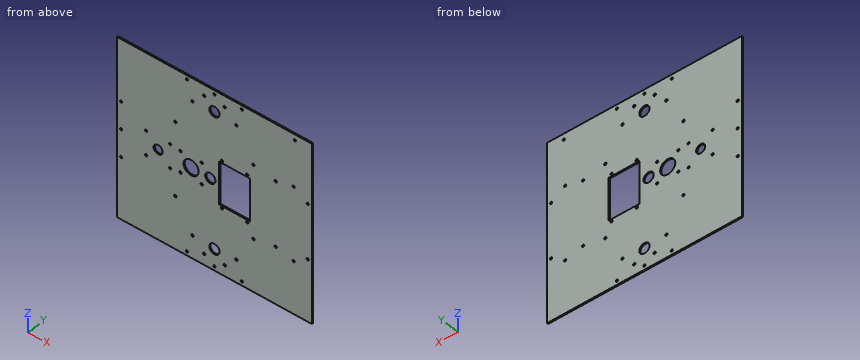
from build123d import *

# Parameters (mm, degrees)
SKETCH_1_W          = 284
SKETCH_1_H          = 260
EXTRUDE_1_DEPTH     = 2
SKETCH_2_R          = 6.65
SKETCH_2_R_2        = 1.6
SKETCH_2_R_3        = 11.05
SKETCH_2_R_4        = 1.75
SKETCH_2_R_5        = 1.65
SKETCH_2_W          = 45
SKETCH_2_H          = 62
CUT_EXTRUDE_1_DEPTH = 10
SKETCH_3_R          = 1.75
CUT_EXTRUDE_2_DEPTH = 10
SKETCH_4_R          = 7.5
CUT_EXTRUDE_3_DEPTH = 10
SKETCH_5_R          = 1.75
CUT_EXTRUDE_4_DEPTH = 4.5


with BuildPart() as part:
    # 草图1 → 凸台-拉伸1 (new body)
    with BuildSketch(Plane(origin=(0, 0, 0), x_dir=(1, 0, 0), z_dir=(0, 1, 0))):
        Rectangle(SKETCH_1_W, SKETCH_1_H)
    extrude(amount=EXTRUDE_1_DEPTH)

    # 草图2 → 切除-拉伸1 (cut)
    with BuildSketch(Plane(origin=(0, 2, 0), x_dir=(1, 0, 0), z_dir=(0, 1, 0))):
        with Locations(Location((-82, 0, 0), (0, 0, 270))):
            Circle(SKETCH_2_R)
        with Locations(Location((-99.536248173, 17.536248173, 0), (0, 0, 270))):
            Circle(SKETCH_2_R_2)
        with Locations(Location((-64.463751827, 17.536248173, 0), (0, 0, 270))):
            Circle(SKETCH_2_R_2)
        with Locations(Location((-64.463751827, -17.536248173, 0), (0, 0, 270))):
            Circle(SKETCH_2_R_2)
        with Locations(Location((-99.536248173, -17.536248173, 0), (0, 0, 270))):
            Circle(SKETCH_2_R_2)
        with Locations(Location((-34, 0, 0), (0, 0, 270))):
            Circle(SKETCH_2_R_3)
        with Locations(Location((-18.5, 15.5, 0), (0, 0, 270))):
            Circle(SKETCH_2_R_4)
        with Locations(Location((-18.5, -15.5, 0), (0, 0, 270))):
            Circle(SKETCH_2_R_4)
        with Locations(Location((-49.5, -15.5, 0), (0, 0, 270))):
            Circle(SKETCH_2_R_4)
        with Locations(Location((-49.5, 15.5, 0), (0, 0, 270))):
            Circle(SKETCH_2_R_4)
        with Locations(Location((-40, 124, 0), (0, 0, 270))):
            Circle(SKETCH_2_R_5)
        with Locations(Location((0, 124, 0), (0, 0, 270))):
            Circle(SKETCH_2_R_5)
        with Locations(Location((40, 124, 0), (0, 0, 270))):
            Circle(SKETCH_2_R_5)
        with Locations(Location((117.5, -121.5, 0), (0, 0, 270))):
            Circle(SKETCH_2_R_5)
        with Locations(Location((40, -124, 0), (0, 0, 270))):
            Circle(SKETCH_2_R_5)
        with Locations(Location((0, -124, 0), (0, 0, 270))):
            Circle(SKETCH_2_R_5)
        with Locations(Location((-40, -124, 0), (0, 0, 270))):
            Circle(SKETCH_2_R_5)
        with Locations(Location((-136, 40, 0), (0, 0, 270))):
            Circle(SKETCH_2_R_5)
        with Locations(Location((-136, -40, 0), (0, 0, 270))):
            Circle(SKETCH_2_R_5)
        with Locations(Location((-136, 0, 0), (0, 0, 270))):
            Circle(SKETCH_2_R_5)
        with Locations(Location((136, 40, 0), (0, 0, 270))):
            Circle(SKETCH_2_R_5)
        with Locations(Location((136, -40, 0), (0, 0, 270))):
            Circle(SKETCH_2_R_5)
        with Locations(Location((115.551101602, -53.6, 0), (0, 0, 270))):
            Circle(SKETCH_2_R_5)
        with Locations(Location((89.320585023, -47.2, 0), (0, 0, 270))):
            Circle(SKETCH_2_R_5)
        with Locations(Location((115.551101602, 53.6, 0), (0, 0, 270))):
            Circle(SKETCH_2_R_5)
        with Locations(Location((89.320585023, 47.2, 0), (0, 0, 270))):
            Circle(SKETCH_2_R_5)
        with Locations(Location((11.15, -34.2, 0), (0, 0, 270))):
            Circle(SKETCH_2_R_4)
        with Locations(Location((47.85, -34.2, 0), (0, 0, 270))):
            Circle(SKETCH_2_R_4)
        with Locations(Location((47.85, 34.2, 0), (0, 0, 270))):
            Circle(SKETCH_2_R_4)
        with Locations(Location((11.15, 34.2, 0), (0, 0, 270))):
            Circle(SKETCH_2_R_4)
        with Locations((29.5, 0)):
            Rectangle(SKETCH_2_W, SKETCH_2_H)
    extrude(amount=-CUT_EXTRUDE_1_DEPTH, mode=Mode.SUBTRACT)

    # 草图3 → 切除-拉伸2 (cut)
    with BuildSketch(Plane(origin=(0, 2, 0), x_dir=(1, 0, 0), z_dir=(0, 1, 0))):
        with Locations(Location((15, -114, 0), (0, 0, 270))):
            Circle(SKETCH_3_R)
        with Locations(Location((-15, -114, 0), (0, 0, 270))):
            Circle(SKETCH_3_R)
        with Locations(Location((15, 114, 0), (0, 0, 270))):
            Circle(SKETCH_3_R)
        with Locations(Location((-15, 114, 0), (0, 0, 270))):
            Circle(SKETCH_3_R)
    extrude(amount=-CUT_EXTRUDE_2_DEPTH, mode=Mode.SUBTRACT)

    # 草图4 → 切除-拉伸3 (cut)
    with BuildSketch(Plane(origin=(0, 2, 0), x_dir=(1, 0, 0), z_dir=(0, 1, 0))):
        with Locations(Location((-6, 0, 0), (0, 0, 270))):
            Circle(SKETCH_4_R)
        with Locations(Location((0, 99, 0), (0, 0, 270))):
            Circle(SKETCH_4_R)
        with Locations(Location((0, -99, 0), (0, 0, 270))):
            Circle(SKETCH_4_R)
    extrude(amount=-CUT_EXTRUDE_3_DEPTH, mode=Mode.SUBTRACT)

    # 草图5 → 切除-拉伸4 (cut)
    with BuildSketch(Plane(origin=(0, 2, 0), x_dir=(1, 0, 0), z_dir=(0, 1, 0))):
        with Locations(Location((57.002701991, 53.5, 0), (0, 0, 270))):
            Circle(SKETCH_5_R)
        with Locations(Location((32.002701991, 96.801270189, 0), (0, 0, 270))):
            Circle(SKETCH_5_R)
        with Locations(Location((-32.002701991, 96.801270189, 0), (0, 0, 270))):
            Circle(SKETCH_5_R)
        with Locations(Location((-57.002701991, 53.5, 0), (0, 0, 270))):
            Circle(SKETCH_5_R)
        with Locations(Location((-57.002701991, -53.5, 0), (0, 0, 270))):
            Circle(SKETCH_5_R)
        with Locations(Location((-32.002701991, -96.801270189, 0), (0, 0, 270))):
            Circle(SKETCH_5_R)
        with Locations(Location((32.002701991, -96.801270189, 0), (0, 0, 270))):
            Circle(SKETCH_5_R)
        with Locations(Location((57.002701991, -53.5, 0), (0, 0, 270))):
            Circle(SKETCH_5_R)
    extrude(amount=-CUT_EXTRUDE_4_DEPTH, mode=Mode.SUBTRACT)


solid = part.part
Source: CAD feature listing. Evaluate the final solid. Frame: model axes, mm. Round coordinates to 2 decimals unless told otherwise and drop trailing zeros. Order: outer loops, then holes, each group sorted by start corner. A loop starts at its lowest first (then second) coordinate and runs counter-clockwise, first axis right, second up. Notation, with made-up numbers: (67, 67) - (85, 67) arc R10 cw to (85, 74) - close; hole circle Ø10 at (85, 42). An arc over 180 degrees is marked (long way). Use a Markdown table: item, result. Add a question column.
1. Line query: probe 1 along Z at (x, y) = (31.5, 0.5); probe 2 along Z at (x, y) = (25, 1.2); probe 3 along X at (y, z) = (0.8, -47.2). Output: solid intervals per line, ascending.
2. First-contact query: pin 1 (2.5 mm diameter, centred on x = 115.55, z = -53.6, fed in from +Y). Flat tip, straight axial feed; report the tip coordinate or a pass-through.
3. Section query B-B (y = 0.55). Give the number of separate pieces and of enclosed holes in the cut face, then the cut area to 3 significant figures.
4. Section query A-A (x = -82). Return the cut outline in (y, z), then the cut area to 3 significant figures.
Derived:
| question | item | result |
|---|---|---|
| 1 | probe 1 | -130 to -98.48, -95.13 to -31, 31 to 95.13, 98.48 to 130 |
| 1 | probe 2 | -130 to -31, 31 to 130 |
| 1 | probe 3 | -142 to 87.67, 90.97 to 142 |
| 2 | pin 1 | through |
| 3 | separate pieces | 1 |
| 3 | enclosed holes | 46 |
| 3 | area | 69,600 mm2 |
| 4 | outline | (0, -130) - (2, -130) - (2, -6.65) - (0, -6.65) - close; (0, 6.65) - (2, 6.65) - (2, 130) - (0, 130) - close |
| 4 | area | 493 mm2 |
